Check sheet for the drawn part. Datum: minimum x, y, z corner. Units: mm. Give positions to 0.01 mm unless a question says otherwise; leave off trailing zeros. Order: outer loops, then holes, each group sorted by start corner. A loop starts at its lowest first (then second) coordinate and runs counter-clockwise, first axis right, second up.
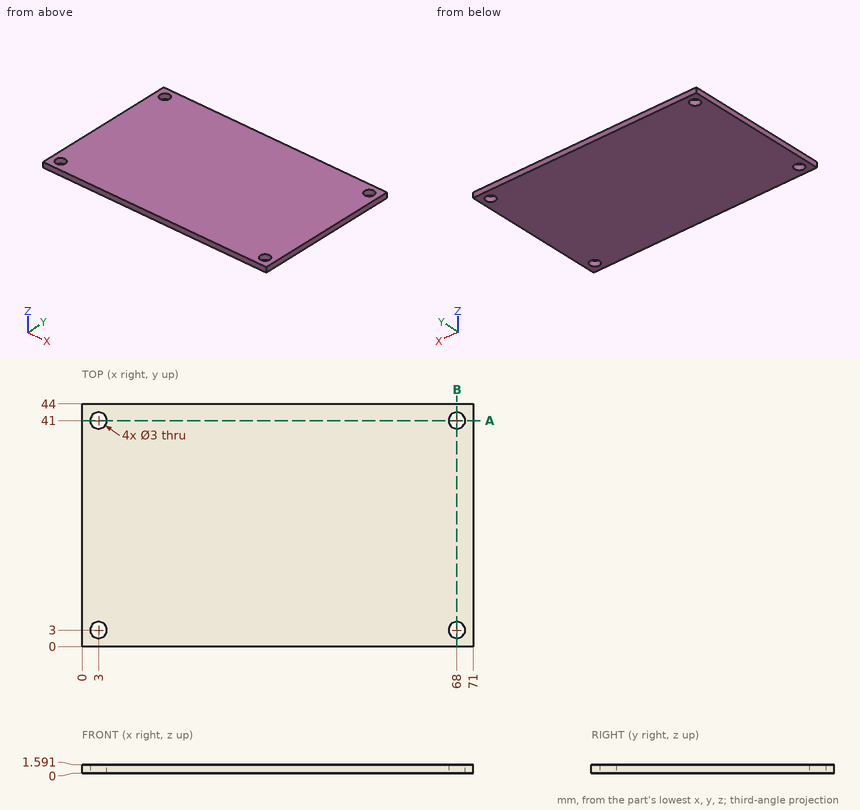
(1) Section check B-B, the plane x = 68. Enter the section's corners in (y, z), then the cut area to 3 significant figures.
Solved:
outline: (0, 0) - (1.5, 0) - (1.5, 1.59) - (0, 1.59) - close; (4.5, 0) - (39.5, 0) - (39.5, 1.59) - (4.5, 1.59) - close; (42.5, 0) - (44, 0) - (44, 1.59) - (42.5, 1.59) - close
area: 60.5 mm2
(2) Section check A-A, the plane y = 41. Enter the section's corners in (x, z), then the cut area to 3 significant figures.
Solved:
outline: (0, 0) - (1.5, 0) - (1.5, 1.59) - (0, 1.59) - close; (4.5, 0) - (66.5, 0) - (66.5, 1.59) - (4.5, 1.59) - close; (69.5, 0) - (71, 0) - (71, 1.59) - (69.5, 1.59) - close
area: 103 mm2
(3) Go/stop test with a flat-tipped pin: pin 1 (3.5 mm diameter, centred on x = 68, y = 41, fed in from -Z). Record where the tip stops, or that it passes through.
Solved:
pin 1: stops at z = 0
(4) Scan lines: line 1 (Y direction, x = 3, z = 0.35); line 2 (X direction, y = 3.5, z = 0.4). Record each from-to range of solid material in increasing order.
Solved:
line 1: y = 0 to 1.5, 4.5 to 39.5, 42.5 to 44
line 2: x = 0 to 1.59, 4.41 to 66.59, 69.41 to 71
